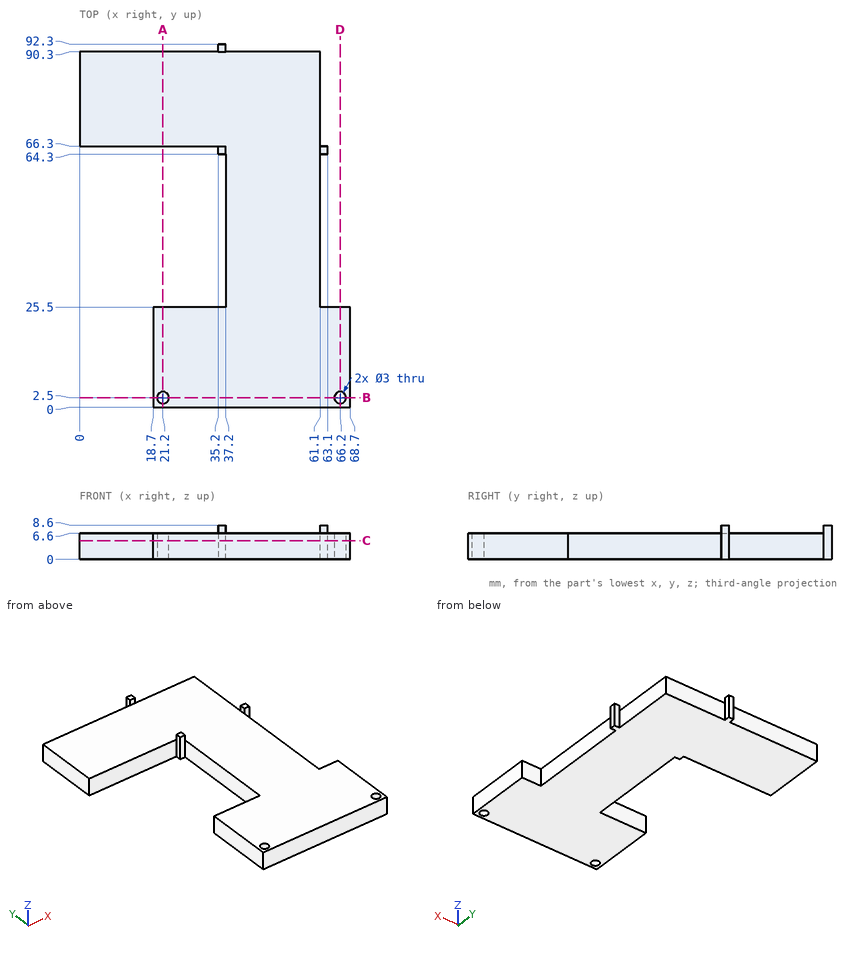
Answer from the drawing. Dimensions are ordinates in mm from the lowest x, y and z of the part. Give positions to 0.01 mm unless a question says otherwise; leave off trailing zeros. Loops run counter-clockwise (first coordinate to the right, second up) from the corner with the lowest first, then second, coordinate; pieces in that order, holes last.
Item 1: Find the intervals of material crossed by line 1 along Y through (x, z) = (21.2, 3.25); line 2 along Y through (x, z) = (66.2, 5); line 3 along Y through (x, z) = (27, 6), in increasing order.
Derived:
line 1: y = 0 to 1, 4 to 25.5, 66.3 to 90.3
line 2: y = 0 to 1, 4 to 25.5
line 3: y = 0 to 25.5, 66.3 to 90.3
Item 2: Each of these flat-tipped pins is pushed along its axis until it touches: pin 1 Ø0.6 at (y, z) = (65.5, 8) entering from -X; pin 2 Ø4 at (y, z) = (46, 6.5) entering from -X; pin 3 Ø2 at (y, z) = (65.5, 7.5) entering from +X; pin 4 Ø1.8 at (x, y) = (66.2, 2.5) entering from -Z. Where does it stop, or does it pass through?
Derived:
pin 1: stops at x = 35.2
pin 2: stops at x = 37.2
pin 3: stops at x = 63.1
pin 4: passes through
Item 3: A cutting plane is placed at A-A (x = 21.2). Give the vertices of the cut face in (y, z), then the cut area to 3 significant figures.
Derived:
outline: (0, 0) - (1, 0) - (1, 6.6) - (0, 6.6) - close; (4, 0) - (25.5, 0) - (25.5, 6.6) - (4, 6.6) - close; (66.3, 0) - (90.3, 0) - (90.3, 6.6) - (66.3, 6.6) - close
area: 307 mm2
Item 4: A cutting plane is placed at B-B (y = 2.5). Give the vertices of the cut face in (x, z).
Derived:
outline: (18.7, 0) - (19.7, 0) - (19.7, 6.6) - (18.7, 6.6) - close; (22.7, 0) - (64.7, 0) - (64.7, 6.6) - (22.7, 6.6) - close; (67.7, 0) - (68.7, 0) - (68.7, 6.6) - (67.7, 6.6) - close
Item 5: A cutting plane is placed at C-C (z = 4.75). Give the vertices of the cut face in (x, y), then the cut area to 3 significant figures.
Derived:
outline: (0, 66.3) - (35.2, 66.3) - (35.2, 64.3) - (37.2, 64.3) - (37.2, 25.5) - (18.7, 25.5) - (18.7, 0) - (68.7, 0) - (68.7, 25.5) - (61.1, 25.5) - (61.1, 64.3) - (63.1, 64.3) - (63.1, 66.3) - (61.1, 66.3) - (61.1, 90.3) - (37.2, 90.3) - (37.2, 92.3) - (35.2, 92.3) - (35.2, 90.3) - (0, 90.3) - close; hole circle Ø3 at (21.2, 2.5); hole circle Ø3 at (66.2, 2.5)
area: 3,710 mm2
Item 6: A cutting plane is placed at D-D (x = 66.2). Give the vertices of the cut face in (y, z), then the cut area to 4 significant figures.
Derived:
outline: (0, 0) - (1, 0) - (1, 6.6) - (0, 6.6) - close; (4, 0) - (25.5, 0) - (25.5, 6.6) - (4, 6.6) - close
area: 148.5 mm2
